Design review of the part built by this model. Coordinates are the model's own, in mm. Face numbers are marked on the shaded views. Round coordinates to 2 decimals unless told otherwise and drop trailing zeros. Write each loop counter-clockwise with the first axis right and the second up, starting at its lowest first coordinate (ties: lowest second). Pieces come first, ordered by that corner, then holes. Notation, with made-up numbers: (21.5, -10.75) -> (31.5, -10.75) arc R10 ccw to (31.5, 1.25) -> close; hole circle Ø2 at (-21.5, 23). An arc over 180 degrees is marked (long way). Write item = value, one per line. Start each with the question number.
Item 1: For pin 1 Ø4 at (x, y) = (-4, 66) entering from -Z, flat-tipped, find the tip position at first contact; note if it passes through.
Item 2: Mouldability with a two-part tool opening along Z and no side actions: class the marked faces 1 and 2 as released by +Z, released by -Z, zero draft, split by the parting line, or undercut.
Item 3: Add section A-A, the plane x = 0. State the section outline as (y, z) points.
Item 4: Add section D-D, the plane x = 4.25. State the section outline as (y, z) points.
Item 5: To check wall thickness, follow L1, parallel to Z at x = 0, y = 27.5; L2, parallel to X at y = 67, z = 1.75; L3, parallel to X at y = 20.5, z = 2. State the ranges of each line that lie inside material, in increasing order.
Item 6: Add section B-B, the plane z = 0. State the section outline as (x, y) points, then the cut area to 4 significant figures.
Item 7: Add section C-C, the plane y = 20.5. State the section outline as (x, z) points, then the cut area to 3 significant figures.
Autodesk Inventor part; units mm, degrees
ref_plane "YZ Plane" through (0, 0, 0) normal (1, 0, 0) x (0, 1, 0)
ref_plane "XZ Plane" through (0, 0, 0) normal (0, 1, 0) x (-1, 0, 0)
ref_plane "XY Plane" through (0, 0, 0) normal (0, 0, 1) x (1, 0, 0)
sketch "Boceto3" plane through (0, 0, 0) normal (0, 1, 0) x (-1, 0, 0)
  circle A0 centre (0, 0) radius 5
  dimension "d10" = 10
extrude "Extrusión2" add sketch "Boceto3" along normal blind 90.7
extrude "Extrusión3" cut sketch "Boceto3" along normal blind 90.7
extrude "Extrusión4" add sketch "Boceto3" along normal blind 90.7
sketch "Boceto4" plane through (0, 90.7, 0) normal (0, 1, 0) x (1, 0, 0)
  point P0 (0, 0)
hole "Agujero2" at (0, 90.7, 0) direction (0, -1, 0) diameter 5 end through all
properties part number "soprye para base bobinas"
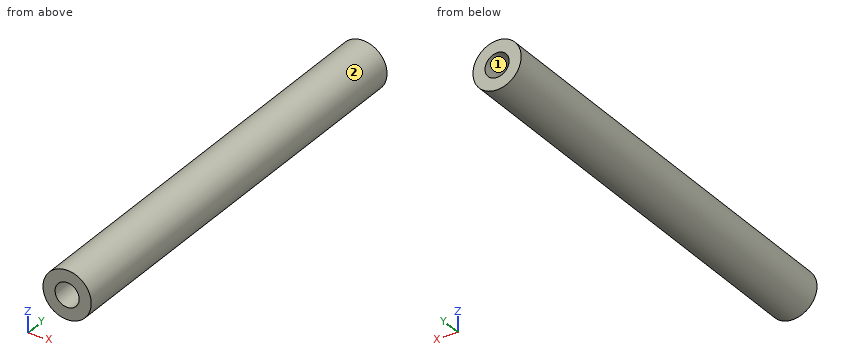
Result set:
q1.pin_1 = -4.58
q2.face_1 = undercut
q2.face_2 = split by the parting line
q3.outline = (0, -5) -> (90.7, -5) -> (90.7, -2.5) -> (0, -2.5) -> close; (0, 2.5) -> (90.7, 2.5) -> (90.7, 5) -> (0, 5) -> close
q4.outline = (0, -2.63) -> (90.7, -2.63) -> (90.7, 2.63) -> (0, 2.63) -> close
q5.L1 = -5 to -2.5, 2.5 to 5
q5.L2 = -4.68 to -1.79, 1.79 to 4.68
q5.L3 = -4.58 to -1.5, 1.5 to 4.58
q6.outline = (-5, 0) -> (-2.5, 0) -> (-2.5, 90.7) -> (-5, 90.7) -> close; (2.5, 0) -> (5, 0) -> (5, 90.7) -> (2.5, 90.7) -> close
q6.area = 453.5 mm²
q7.outline = circle Ø10 at (0, 0); hole circle Ø5 at (0, 0)
q7.area = 58.9 mm²
